Could you check a few things on this drawing? It's one solid part, dimensions in mm from its lowest x, y, z. A direction names the side the tool comes from. Give positions to 0.01 mm unless a question says otherwise; leave off trailing zeros. Order: outer loops, then holes, each group sorted by start corner. A loop starts at its lowest first (then second) coordinate and runs counter-clockwise, first axis right, second up. Notation, with made-up numbers: M 88,89 L 132,89 A17 ccw 132,93 Z; hole C 37,47.25 d4. An arc over 180 degrees is marked long. One line per item, written item: value. Start each with the question number.
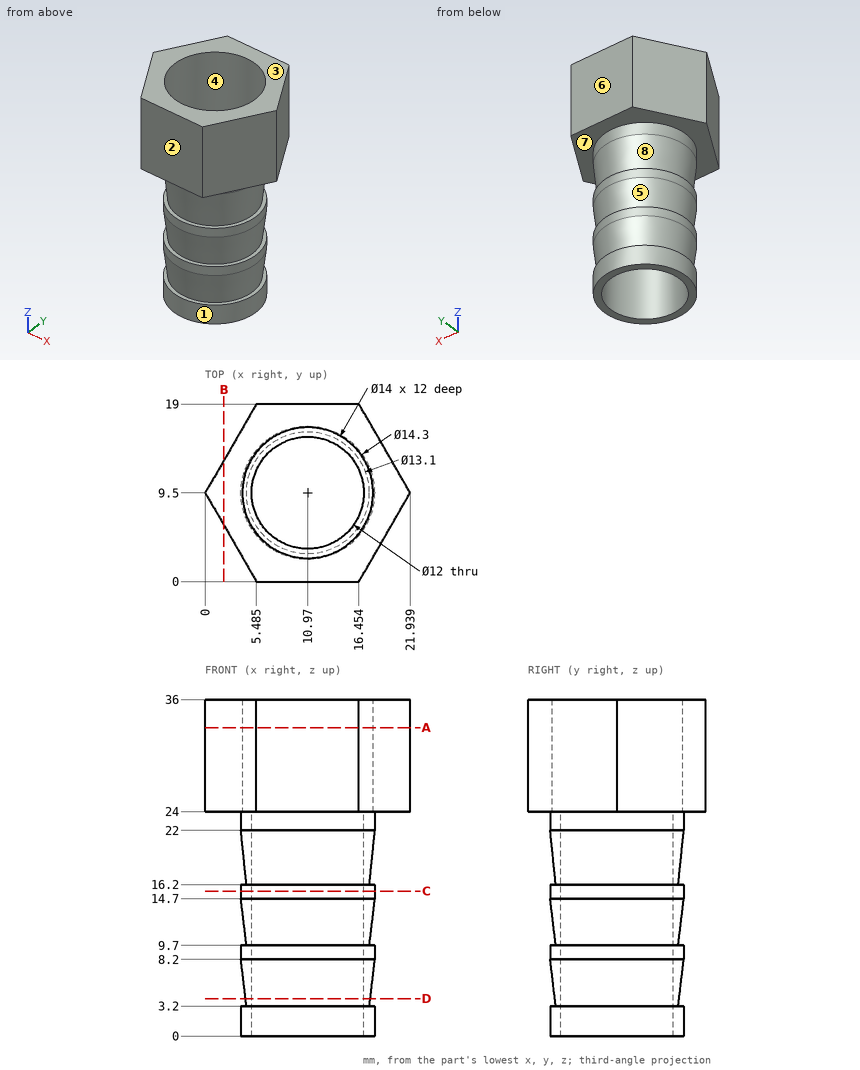
Item 1: Will these pins go through, and if not, where does the flat tip stop? P1, Ø12, axis at x = 7, z = 9, coming from the -Y side; P2, Ø5, axis at y = 17, z = 19, coming from the +X side (1 decimal); P3, Ø9.5, axis at x = 7, y = 8, coming from the -Z side; P4, Ø7, axis at x = 10, y = 11, coming from the +Z side.
Item 2: I want a section at A-A on z = 33. Write out the boundary of the cut face in (x, y) (1 decimal), plus the area to 3 significant figures.
Item 3: I want a section at D-D on z = 4. Write out the boundary of the cut face in (x, y) (1 decimal).
Item 4: For the marked faces 1, 2, 3, 4 and 5, which set-ups out of +Z, -Z, +X, -X, +Y, -Y let a thin tool reach every point of the face, with its end or its side?
Item 5: We'd pull the mould along Z, two halves only. Please class the marked faces 6, 7 and 8: +Z half, -Z half, draft (parallel to the pull), parting line (faces both ways), or undercut.
Item 6: I want a section at B-B on x = 2. Write out the boundary of the cut face in (y, z) (1 decimal).
Item 7: Please list where these lines run through material, in increasing order: probe 1 along Z at (x, y) = (2.5, 13); probe 2 along Y at (x, z) = (15.75, 6) (1 decimal); probe 3 along X at (y, z) = (9.5, 5) (1 decimal). Write a range as [from, to].
Item 8: I want a section at C-C on z = 15.5. Write out the boundary of the cut face in (x, y).
Answer below:
1. P1: stops at y = 2.35
1. P2: stops at x = 15.7
1. P3: stops at z = 0
1. P4: passes through
2. outline: M 0,9.5 L 5.5,0 L 16.5,0 L 21.9,9.5 L 16.5,19 L 5.5,19 Z; hole C 11,9.5 d14
2. area: 159 mm²
3. outline: C 11,9.5 d13.3; hole C 11,9.5 d12
4. face 1: -Z
4. face 2: +Z, -Z, +X, -X, -Y
4. face 3: +Z, +X, -X, +Y, -Y
4. face 4: +Z
4. face 5: none
5. face 6: draft
5. face 7: -Z half
5. face 8: undercut
6. outline: M 6,24 L 13,24 L 13,36 L 6,36 Z
7. probe 1: z = [24, 36]
7. probe 2: y = [4.5, 5.9], [13.1, 14.5]
7. probe 3: x = [4.2, 5], [17, 17.7]
8. outline: C 10.97,9.5 d14.3; hole C 10.97,9.5 d12
